```python
from build123d import *

# Parameters (mm, degrees)
TRAY_SECTION_DEPTH         = 292
REAR_WALL_DEPTH            = 90
FRONT_WALL_DEPTH           = 90
EAR_RELIEF_SKETCH_W        = 17
EAR_RELIEF_SKETCH_H        = 4.3
EAR_RELIEF_SKETCH_W_2      = 21
EAR_RELIEFS_DEPTH          = 26.4
MOUNTING_EAR_SKETCH_W      = 16
MOUNTING_EAR_SKETCH_H      = 15.2
MOUNTING_EAR_SKETCH_W_2    = 20
MOUNTING_EARS_DEPTH        = 2
TRAY_HOLE_SKETCH_R         = 1.7
TRAY_HOLE_SKETCH_R_2       = 3.3
TRAY_HOLES_AND_SLOTS_DEPTH = 2.4
CLAMP_CLEARANCE_SKETCH_W   = 33
CLAMP_CLEARANCE_SKETCH_H   = 14.7
CLAMP_CLEARANCE_DEPTH      = 130


with BuildPart() as part:
    # Tray Section Sketch → Tray Section (new body)
    with BuildSketch(Plane(origin=(-153.5, 0, 0), x_dir=(0, 0, -1), z_dir=(1, 0, 0))):
        with BuildLine():
            Line((-144, -49), (-122, -49))
            ThreePointArc((-122, -49), (-119.171572875, -47.828427125), (-118, -45))
            Line((-118, -45), (-118, 45))
            ThreePointArc((-118, 45), (-119.171572875, 47.828427125), (-122, 49))
            Line((-122, 49), (-144, 49))
            Line((-144, 49), (-144, 47))
            Line((-144, 47), (-122, 47))
            ThreePointArc((-122, 47), (-120.585786438, 46.414213562), (-120, 45))
            Line((-120, 45), (-120, -45))
            ThreePointArc((-120, -45), (-120.585786438, -46.414213562), (-122, -47))
            Line((-122, -47), (-144, -47))
            Line((-144, -47), (-144, -49))
        make_face()
    extrude(amount=TRAY_SECTION_DEPTH)

    # Rear Wall Sketch → Rear Wall (add)
    with BuildSketch(Plane(origin=(0, -45, 0), x_dir=(-1, 0, 0), z_dir=(0, -1, 0))):
        with BuildLine():
            Line((157.5, -122), (157.5, -144))
            Line((157.5, -144), (155.5, -144))
            Line((155.5, -144), (155.5, -122))
            ThreePointArc((155.5, -122), (154.914213562, -120.585786438), (153.5, -120))
            Line((153.5, -120), (153.5, -118))
            ThreePointArc((153.5, -118), (156.328427125, -119.171572875), (157.5, -122))
        make_face()
    extrude(amount=-REAR_WALL_DEPTH)

    # Front Wall Sketch → Front Wall (add)
    with BuildSketch(Plane(origin=(0, -45, 0), x_dir=(-1, 0, 0), z_dir=(0, -1, 0))):
        with BuildLine():
            Line((-142.5, -122), (-142.5, -144))
            Line((-142.5, -144), (-140.5, -144))
            Line((-140.5, -144), (-140.5, -122))
            ThreePointArc((-140.5, -122), (-139.914213562, -120.585786438), (-138.5, -120))
            Line((-138.5, -120), (-138.5, -118))
            ThreePointArc((-138.5, -118), (-141.328427125, -119.171572875), (-142.5, -122))
        make_face()
    extrude(amount=-FRONT_WALL_DEPTH)

    # Ear Relief Sketch → Ear Reliefs (cut)
    with BuildSketch(Plane.XY.offset(117.8)):
        with Locations((-90, -47.05)):
            Rectangle(EAR_RELIEF_SKETCH_W, EAR_RELIEF_SKETCH_H)
        with Locations((-90, 47.05)):
            Rectangle(EAR_RELIEF_SKETCH_W, EAR_RELIEF_SKETCH_H)
        with Locations((75, -47.05)):
            Rectangle(EAR_RELIEF_SKETCH_W, EAR_RELIEF_SKETCH_H)
        with Locations((75, 47.05)):
            Rectangle(EAR_RELIEF_SKETCH_W, EAR_RELIEF_SKETCH_H)
        with Locations((-18, -47.05)):
            Rectangle(EAR_RELIEF_SKETCH_W_2, EAR_RELIEF_SKETCH_H)
        with Locations((-18, 47.05)):
            Rectangle(EAR_RELIEF_SKETCH_W_2, EAR_RELIEF_SKETCH_H)
    extrude(amount=EAR_RELIEFS_DEPTH, mode=Mode.SUBTRACT)

    # Mounting Ear Sketch → Mounting Ears (add)
    with BuildSketch(Plane.XY.offset(118)):
        with Locations((-90, -52.4)):
            Rectangle(MOUNTING_EAR_SKETCH_W, MOUNTING_EAR_SKETCH_H)
        with Locations((-90, 52.4)):
            Rectangle(MOUNTING_EAR_SKETCH_W, MOUNTING_EAR_SKETCH_H)
        with Locations((75, -52.4)):
            Rectangle(MOUNTING_EAR_SKETCH_W, MOUNTING_EAR_SKETCH_H)
        with Locations((75, 52.4)):
            Rectangle(MOUNTING_EAR_SKETCH_W, MOUNTING_EAR_SKETCH_H)
        with Locations((-18, -52.4)):
            Rectangle(MOUNTING_EAR_SKETCH_W_2, MOUNTING_EAR_SKETCH_H)
        with Locations((-18, 52.4)):
            Rectangle(MOUNTING_EAR_SKETCH_W_2, MOUNTING_EAR_SKETCH_H)
    extrude(amount=MOUNTING_EARS_DEPTH)

    # Tray Hole Sketch → Tray Holes and Slots (cut)
    with BuildSketch(Plane.XY.offset(117.8)):
        with Locations(Location((-90, -51.5, 0), (0, 0, 180))):
            Circle(TRAY_HOLE_SKETCH_R)
        with Locations(Location((-90, 51.5, 0), (0, 0, 180))):
            Circle(TRAY_HOLE_SKETCH_R)
        with Locations(Location((75, -51.5, 0), (0, 0, 180))):
            Circle(TRAY_HOLE_SKETCH_R)
        with Locations(Location((75, 51.5, 0), (0, 0, 180))):
            Circle(TRAY_HOLE_SKETCH_R)
        with Locations(Location((-18, -51.5, 0), (0, 0, 180))):
            Circle(TRAY_HOLE_SKETCH_R_2)
        with Locations(Location((-18, 51.5, 0), (0, 0, 180))):
            Circle(TRAY_HOLE_SKETCH_R_2)
        with BuildLine():
            Line((-151.5, -1.7), (-137.5, -1.7))
            ThreePointArc((-137.5, -1.7), (-135.8, 0), (-137.5, 1.7))
            Line((-137.5, 1.7), (-151.5, 1.7))
            ThreePointArc((-151.5, 1.7), (-153.2, 0), (-151.5, -1.7))
        make_face()
        with BuildLine():
            Line((122.5, -1.7), (136.5, -1.7))
            ThreePointArc((136.5, -1.7), (138.2, 0), (136.5, 1.7))
            Line((136.5, 1.7), (122.5, 1.7))
            ThreePointArc((122.5, 1.7), (120.8, 0), (122.5, -1.7))
        make_face()
    extrude(amount=TRAY_HOLES_AND_SLOTS_DEPTH, mode=Mode.SUBTRACT)

    # Clamp Clearance Sketch → Clamp Clearance (cut)
    with BuildSketch(Plane(origin=(0, -65, 0), x_dir=(-1, 0, 0), z_dir=(0, -1, 0))):
        with Locations((7.5, -136.85)):
            Rectangle(CLAMP_CLEARANCE_SKETCH_W, CLAMP_CLEARANCE_SKETCH_H)
    extrude(amount=-CLAMP_CLEARANCE_DEPTH, mode=Mode.SUBTRACT)


solid = part.part
```
For this review, take the finished solid that the model builds, in its own axes (mm). A direction names the side the tool comes from. Round coordinates to 2 decimals unless told otherwise and drop trailing zeros. Order: outer loops, then holes, each group sorted by start corner. A loop starts at its lowest first (then second) coordinate and runs counter-clockwise, first axis right, second up. Notation, with made-up numbers: (-14.75, 5.5) -> (13.25, 5.5) arc R28 ccw to (13.25, 35.5) -> close; hole circle Ø5 at (41, 12.5). An arc over 180 degrees is marked (long way). Use a Markdown table: item, result.
Item 1: Take a section at B-B (y = -30.5). State the section outline as (x, z) points.
Resolved:
| item | result |
|---|---|
| outline | (-157.5, 122) arc R4 ccw to (-153.5, 118) -> (138.5, 118) arc R4 ccw to (142.5, 122) -> (142.5, 144) -> (140.5, 144) -> (140.5, 122) arc R2 cw to (138.5, 120) -> (-153.5, 120) arc R2 cw to (-155.5, 122) -> (-155.5, 144) -> (-157.5, 144) -> close |
Item 2: For line 1 along Y through (x, z) = (-90, 119.5); line 2 along Y through (x, z) = (-18, 119.5); line 3 along X through (y, z) = (-15, 122.75), list the stretches that pass through material, from the lowest coordinate up. Write a range as [from, to].
Resolved:
| item | result |
|---|---|
| line 1 | y = [-60, -53.2], [-49.8, 49.8], [53.2, 60] |
| line 2 | y = [-60, -54.8], [-48.2, 48.2], [54.8, 60] |
| line 3 | x = [-157.5, -155.5], [140.5, 142.5] |
Item 3: Take a section at C-C (z = 125.25). State how many separate pieces and enclosed holes the cut face has, plus the area to 3 significant figures.
Resolved:
| item | result |
|---|---|
| separate pieces | 10 |
| enclosed holes | 0 |
| area | 1,310 mm² |
Item 4: For pin 1 (2 mm diameter, centred on x = -53.5, y = 36, fed in from +Z); pin 2 (2 mm diameter, centred on y = 54.5, z = 119, fed in from -X); pin 3 (3.5 mm diameter, centred on y = -47.5, z = 130, fed in from +X), all flat-tipped, find the tip position at first contact; note any pin that passes through.
Resolved:
| item | result |
|---|---|
| pin 1 | stops at z = 120 |
| pin 2 | stops at x = -98 |
| pin 3 | stops at x = 138.5 |
Item 5: Take a section at D-D (x = 46.5). State the section outline as (y, z) points.
Resolved:
| item | result |
|---|---|
| outline | (-49, 122) arc R4 ccw to (-45, 118) -> (45, 118) arc R4 ccw to (49, 122) -> (49, 144) -> (47, 144) -> (47, 122) arc R2 cw to (45, 120) -> (-45, 120) arc R2 cw to (-47, 122) -> (-47, 144) -> (-49, 144) -> close |
Item 6: Draft analysis for pull direction Y (two halves, no side actions). For faces 6 (the flat face through (-55, -47, 133)), 7 (the flat face through (-55, 47, 133)), 8 (the flat face through (37, 49, 133)), 9 (the flat face through (-55, -49, 133)), state which applies: +Y half, -Y half, draft (parallel to the pull), parting line (faces both ways), or undercut.
Resolved:
| item | result |
|---|---|
| face 6 | undercut |
| face 7 | undercut |
| face 8 | +Y half |
| face 9 | -Y half |
Item 7: Machinability: for faces 1 (the flat face through (37, -49, 133)), 2 (the flat face through (140.5, -1, 133)), 3 (the flat face through (-10, 1, 120)), 4 (the flat face through (-10, 1, 118)), 5 (the flat face through (-126, 47, 133)), which of the approach directions +Z, -Z, +X, -X, +Y, -Y give a long, thin tool a straight path to every point of the face, cutting with its end or side? Answer none if there is none.
Resolved:
| item | result |
|---|---|
| face 1 | +Z, -Z, +X, -X, -Y |
| face 2 | +Z, +Y, -Y |
| face 3 | +Z |
| face 4 | -Z, +X, -X, +Y, -Y |
| face 5 | +Z, +X, -X |
Item 8: Take a section at A-A (x = -18). State the section outline as (y, z) points.
Resolved:
| item | result |
|---|---|
| outline | (-60, 118) -> (-54.8, 118) -> (-54.8, 120) -> (-60, 120) -> close; (-48.2, 118) -> (48.2, 118) -> (48.2, 120) -> (-48.2, 120) -> close; (54.8, 118) -> (60, 118) -> (60, 120) -> (54.8, 120) -> close |
